The drawing under review shows one solid part. Ordinate dimensions are in mm from its lowest x, y, z. A direction names the side the tool comes from. Round coordinates to 2 decimals unless told otherwise and drop trailing zeros. Order: outer loops, then holes, each group sorted by start corner. A loop starts at its lowest first (then second) coordinate and runs counter-clockwise, first axis right, second up. Notation, with made-up numbers: M 85.5,-34 L 139.5,-34 A4 ccw 139.5,-30 Z; hole C 57,39 d6. An arc over 180 degrees is marked long. Use a Markdown table: item, result.
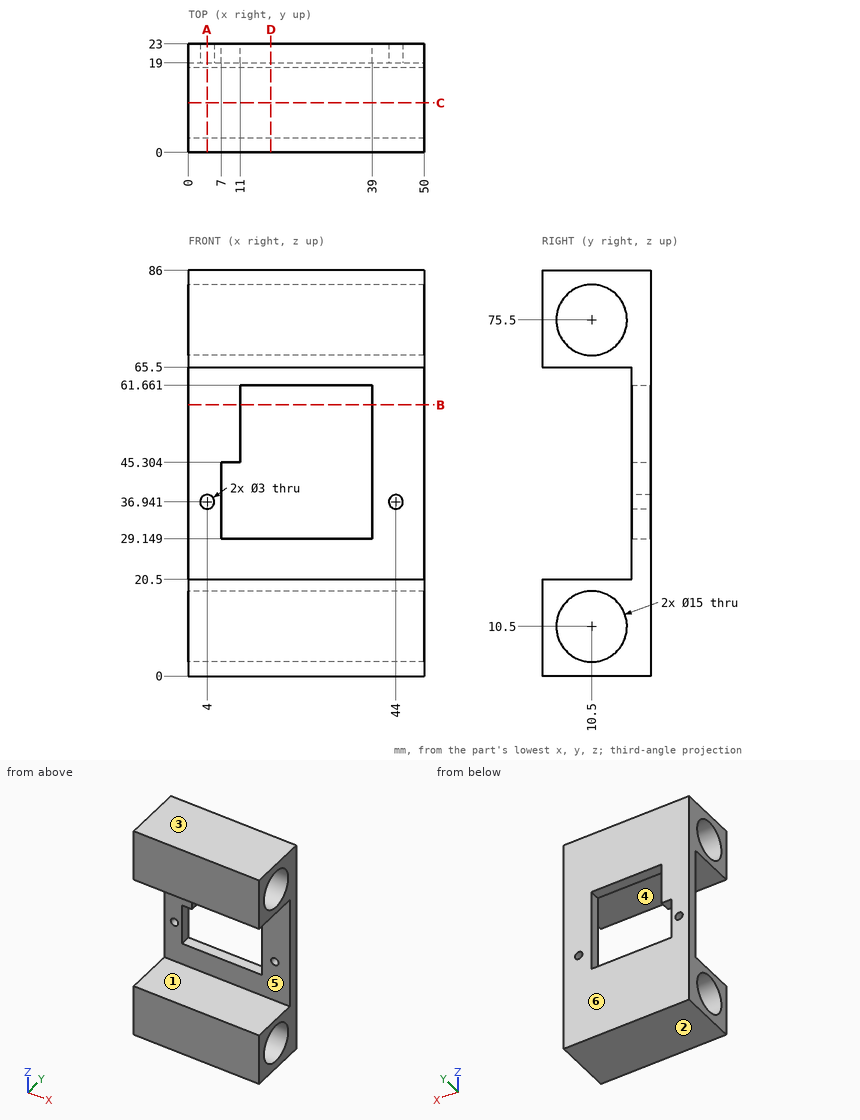
Q1. Add section B-B (z = 57.5). Write out the cut boundary in (x, y).
Determined:
| item | result |
|---|---|
| outline | M 0,19 L 11,19 L 11,23 L 0,23 Z; M 39,19 L 50,19 L 50,23 L 39,23 Z |
Q2. Add section A-A (x = 4). Write out the cut boundary in (y, z).
Determined:
| item | result |
|---|---|
| outline | M 0,0 L 23,0 L 23,35.44 L 19,35.44 L 19,20.5 L 0,20.5 Z; M 0,65.5 L 19,65.5 L 19,38.44 L 23,38.44 L 23,86 L 0,86 Z; hole C 10.5,10.5 d15; hole C 10.5,75.5 d15 |
Q3. Add section D-D (x = 17.5). Write out the cut boundary in (y, z).
Determined:
| item | result |
|---|---|
| outline | M 0,0 L 23,0 L 23,29.15 L 19,29.15 L 19,20.5 L 0,20.5 Z; M 0,65.5 L 19,65.5 L 19,61.66 L 23,61.66 L 23,86 L 0,86 Z; hole C 10.5,10.5 d15; hole C 10.5,75.5 d15 |
Q4. Draft analysis for pull direction Z (two halves, no side actions). For the marked faces 1, 2, 3 and 4, state which applies: pulls with the +Z half, pulls with the -Z half, needs draft (parallel to the pull), parting line crosses it, or undercut.
Determined:
| item | result |
|---|---|
| face 1 | undercut |
| face 2 | pulls with the -Z half |
| face 3 | pulls with the +Z half |
| face 4 | undercut |
Q5. Clearance check with flat-ended pins moving along their axes: pin 1 (1.2 mm diameter, centred on x = 9.5, y = 20.5, fed in from -Z); pin 2 (3 mm diameter, centred on x = 37.5, z = 61.5, fed in from -Y). State where each tip first meets the part, or that it passes through.
Determined:
| item | result |
|---|---|
| pin 1 | stops at z = 0 |
| pin 2 | stops at y = 19 |
Q6. Wall thickness on line 1 along X through (y, z) = (20.5, 57); line 2 along Z through (x, y) = (25.5, 18.5); line 3 along Z through (x, y) = (18.5, 9): over which ranges is each line inside the solid? List them lowest first. Write a range as [from, to].
Determined:
| item | result |
|---|---|
| line 1 | x = [0, 11], [39, 50] |
| line 2 | z = [0, 20.5], [65.5, 86] |
| line 3 | z = [0, 3.15], [17.85, 20.5], [65.5, 68.15], [82.85, 86] |
Q7. Machinability: for the marked faces 5 and 6, which of the approach directions +Z, -Z, +X, -X, +Y, -Y give a long, thin tool a straight path to every point of the face, cutting with its end or side? Answer none if there is none.
Determined:
| item | result |
|---|---|
| face 5 | +X, -X, -Y |
| face 6 | +Z, -Z, +X, -X, +Y |
Q8. Add section C-C (y = 10.5). Write out the cut boundary in (x, z), then the cut area to 3 significant figures.
Determined:
| item | result |
|---|---|
| outline | M 0,0 L 50,0 L 50,3 L 0,3 Z; M 0,18 L 50,18 L 50,20.5 L 0,20.5 Z; M 0,65.5 L 50,65.5 L 50,68 L 0,68 Z; M 0,83 L 50,83 L 50,86 L 0,86 Z |
| area | 550 mm^2 |
